Could you check a few things on this model? Use its own coordinates, in mm. Face numbers are marked on the shaded views. A direction names the side the tool comes from. Give positions to 0.01 mm unless a question says otherwise; leave off trailing zeros. Write each loop counter-clockwise with the first axis right and the second up, starting at its lowest first coordinate (ties: lowest second). Pieces come first, ordered by that corner, then holes. Notation, with made-up numbers: M 52.5,44 L 104.5,44 A36 ccw 104.5,81 Z; hole C -6,57 d5. An arc over 180 degrees is marked long. One line per item, written item: value.
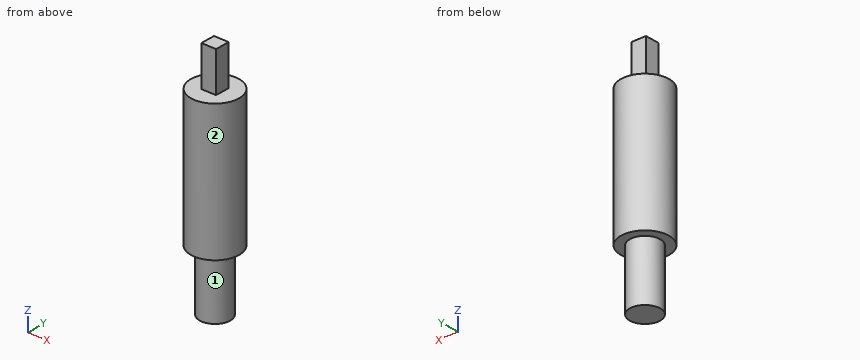
```python
from build123d import *

# Parameters (mm, degrees)
SKETCH1_W      = 3.7
SKETCH1_H      = 3.7
EXTRUDE1_DEPTH = 10
SKETCH2_R      = 6
EXTRUDE2_DEPTH = 34
SKETCH3_R      = 3.8
EXTRUDE3_DEPTH = 15


with BuildPart() as part:
    # Sketch1 → Extrude1 (new body)
    with BuildSketch(Plane.XY):
        Rectangle(SKETCH1_W, SKETCH1_H)
    extrude(amount=EXTRUDE1_DEPTH)

    # Sketch2 → Extrude2 (add)
    with BuildSketch(Plane(origin=(0, 0, 0), x_dir=(-1, 0, 0), z_dir=(0, 0, -1))):
        Circle(SKETCH2_R)
    extrude(amount=EXTRUDE2_DEPTH)

    # Sketch3 → Extrude3 (add)
    with BuildSketch(Plane(origin=(0, 0, -34), x_dir=(-1, 0, 0), z_dir=(0, 0, -1))):
        Circle(SKETCH3_R)
    extrude(amount=EXTRUDE3_DEPTH)


solid = part.part
```
1) If we section it at D-D, the plane x = -2.5: Write out the boundary of the cut face in (y, z), then the cut area to 3 significant figures.
Outcome:
outline: M -5.45,-34 L -2.86,-34 L -2.86,-49 L 2.86,-49 L 2.86,-34 L 5.45,-34 L 5.45,0 L -5.45,0 Z
area: 457 mm^2
2) I'm going to push flat-ended pins straight in: pin 1 (6 mm diameter, centred on y = 3.5, z = -37.5, fed in from +X); pin 2 (1.8 mm diameter, centred on x = -0.5, z = 6.5, fed in from -Y); pin 3 (3 mm diameter, centred on y = 3.5, z = 3, fed in from +X); pin 4 (1 mm diameter, centred on x = -4, z = -5, fed in from +Y). Where does each tip first touch, or does it pass through?
Outcome:
pin 1: stops at x = 3.77
pin 2: stops at y = -1.85
pin 3: passes through
pin 4: stops at y = 4.87
3) Please list where these lines run through material, in increasing order: L1, parallel to Z at x = -2.5, y = 1.5; L2, parallel to Z at x = -3, y = 2.5; L3, parallel to X at y = -1.75, z = 7. Write a range as from..to.
Outcome:
L1: z = -49..0
L2: z = -34..0
L3: x = -1.85..1.85
4) If we section it at C-C, the plane z = -25: Write out the boundary of the cut face in (x, y), then the cut area to 3 significant figures.
Outcome:
outline: C 0,0 d12
area: 113 mm^2
5) If we section it at A-A, the plane y = 0: Write out the boundary of the cut face in (x, z), then the cut area to 3 significant figures.
Outcome:
outline: M -6,-34 L -3.8,-34 L -3.8,-49 L 3.8,-49 L 3.8,-34 L 6,-34 L 6,0 L 1.85,0 L 1.85,10 L -1.85,10 L -1.85,0 L -6,0 Z
area: 559 mm^2
6) On a 3-axis mill with a long thin cutter (end or side, diameter ignored), from which of +Z, -Z, +X, -X, +Y, -Y can I reach the whole of each face in a straight line? I mean the marked faces 1 and 2. Say none if no direction works.
Outcome:
face 1: -Z
face 2: +Z, -Z
